Geometry check sheet. Reference: the model listing, model coordinates, mm. A direction names the side the tool comes from. Round coordinates to 2 decimals unless told otherwise and drop trailing zeros. Write each loop counter-clockwise with the first axis right and the second up, starting at its lowest first coordinate (ties: lowest second). Pieces come first, ordered by that corner, then holes. Notation, with made-up numbers: M 72.25,79.5 L 104.25,79.5 A17 ccw 104.25,85.5 Z; hole C 60.5,-9.5 d3. An arc over 180 degrees is marked long. Put each result on its own line as item: value. Start each with the question number.
(1) Material ranges on probe 1 along Y at (x, z) = (6.75, 1.5); probe 2 along Y at (x, z) = (6.25, -4.5); probe 3 along X at (y, z) = (1, -1), recorded low to high.
(2) Section check C-C on x = 6.25. Record the cut outline in (y, z) (3 decimals), then the cut area to 3 significant figures.
(3) Mould release check, pull along Y, two halves, no side actions. Record for faces 1 (the cylindrical face through (7.817, 2.989, -0.002)), 2 (the flat face through (3.9, 7, 2)), 3 (the flat face through (7, 0, -1)): pulls with the +Y half, pulls with the -Y half, needs draft (parallel to the pull), parting line crosses it, or undercut.
(4) Section check B-B on z = -2.5. Record the cut outline in (x, y) (3 decimals), then the cut area to 3 significant figures.
(5) Section check D-D on y = 5.5. Record the cut outline in (x, z) (3 decimals).
(6) Tool access check on faces 4 (the flat face through (1, 7, 0)), 5 (the flat face through (7, 7, 4.675)), 6 (the flat face through (3, 7, -1.1)), 7 (the flat face through (2.75, 7, -5)), 8 (the flat face through (7, 15, -1)). Record the directions out of +Z, -Z, +X, -X, +Y, -Y that give a thin tool (end or side, any length) a straight path to the whole face; none if there is none.
(7) Gauge pin test, flat ends, axial feed: pin 1 (4 mm diameter, centred on x = 8, y = 10, fed in from -Z); pin 2 (0.6 mm diameter, centred on y = 7.5, z = -5, fed in from +X); pin 3 (1.4 mm diameter, centred on x = 1, y = 9, fed in from +Z). Record the tip position at first contact, or that the pin passes through.
(8) Section check A-A on y = 11.25. Record the cut outline in (x, z) (3 decimals), then the cut area to 3 significant figures.
from build123d import *

# Parameters (mm, degrees)
SKETCH1_W           = 2.75
SKETCH1_H           = 5.65
SKETCH1_W_2         = 1.15
SKETCH1_H_2         = 1.725
BOSS_EXTRUDE1_DEPTH = 15
SKETCH2_R           = 1.25
CUT_EXTRUDE1_DEPTH  = 21.710157532


with BuildPart() as part:
    # Sketch1 → Boss-Extrude1 (new body)
    with BuildSketch(Plane(origin=(0, 0, 0), x_dir=(1, 0, 0), z_dir=(0, 1, 0))):
        with Locations((1.375, 2.825)):
            Rectangle(SKETCH1_W, SKETCH1_H)
        with Locations((3.325, 3.6875)):
            Rectangle(SKETCH1_W_2, SKETCH1_H_2)
        with Locations((3.325, 1.9625)):
            Rectangle(SKETCH1_W_2, SKETCH1_H_2)
        Polygon((10.9, -4.675), (10.9, 4.55), (3.9, 4.55), (3.9, 2.825), (3.9, -4.675), align=None)
    extrude(amount=BOSS_EXTRUDE1_DEPTH)

    # Sketch2 → Cut-Extrude1 (cut, through all)
    with BuildSketch(Plane(origin=(0, 0, -4.55), x_dir=(-1, 0, 0), z_dir=(0, 0, -1))):
        with Locations((-6.825, 11.25)):
            Circle(SKETCH2_R)
        with Locations((-6.825, 3.75)):
            Circle(SKETCH2_R)
    extrude(amount=-CUT_EXTRUDE1_DEPTH, mode=Mode.SUBTRACT)


solid = part.part
Answers follow:
1. probe 1: y = 0 to 2.5, 5 to 10, 12.5 to 15
1. probe 2: y = 0 to 2.64, 4.86 to 10.14, 12.36 to 15
1. probe 3: x = 0 to 2.75, 3.9 to 10.9
2. outline: M 0,-4.55 L 2.64,-4.55 L 2.64,4.675 L 0,4.675 Z; M 4.86,-4.55 L 10.14,-4.55 L 10.14,4.675 L 4.86,4.675 Z; M 12.36,-4.55 L 15,-4.55 L 15,4.675 L 12.36,4.675 Z
2. area: 97.4 mm^2
3. face 1: undercut
3. face 2: needs draft
3. face 3: pulls with the -Y half
4. outline: M 0,0 L 10.9,0 L 10.9,15 L 0,15 Z; hole C 6.825,3.75 d2.5; hole C 6.825,11.25 d2.5
4. area: 154 mm^2
5. outline: M 0,-5.65 L 2.75,-5.65 L 2.75,-4.55 L 10.9,-4.55 L 10.9,4.675 L 3.9,4.675 L 3.9,-1.1 L 2.75,-1.1 L 2.75,0 L 0,0 Z
6. face 4: +Z, -X, +Y, -Y
6. face 5: +Z, +X, -X, +Y, -Y
6. face 6: +Z, +Y, -Y
6. face 7: -Z, +X, +Y, -Y
6. face 8: +Z, -Z, +X, -X, +Y
7. pin 1: stops at z = -4.55
7. pin 2: stops at x = 2.75
7. pin 3: stops at z = 0
8. outline: M 0,-5.65 L 2.75,-5.65 L 2.75,-4.55 L 5.575,-4.55 L 5.575,4.675 L 3.9,4.675 L 3.9,-1.1 L 2.75,-1.1 L 2.75,0 L 0,0 Z; M 8.075,-4.55 L 10.9,-4.55 L 10.9,4.675 L 8.075,4.675 Z
8. area: 61.0 mm^2
